The model under review builds one solid part; all positions refer to its coordinate system, in mm. Give positions to 0.01 mm unless a question says otherwise; leave off trailing zeros. Write each loop counter-clockwise with the first axis right and the second up, starting at its lowest first coordinate (ties: lowest second). Pieces come first, ordered by that corner, then holes.
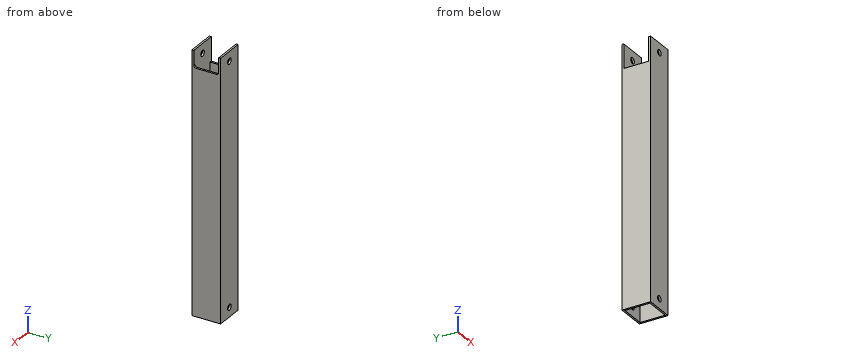
Solid Edge part; units mm, degrees
sketch "Sketch1" plane through (0, 0, 0) normal (0, 0, 1) x (1, 0, 0)
  line L0 (-81.6266, 67.336) -> (-21.6266, 67.336)
  line L1 (-21.6266, 67.336) -> (-21.6266, 127.336)
  line L2 (-21.6266, 127.336) -> (-81.6266, 127.336)
  line L3 (-81.6266, 127.336) -> (-81.6266, 67.336)
  line L4 (-77.6266, 71.336) -> (-25.6266, 71.336)
  line L5 (-25.6266, 71.336) -> (-25.6266, 123.336)
  line L6 (-25.6266, 123.336) -> (-77.6266, 123.336)
  line L7 (-77.6266, 123.336) -> (-77.6266, 71.336)
  dimension "D1" = 21.6266
  dimension "D2" = 81.6266
extrude "Protrusion1" add sketch "Sketch1" along normal blind 540
sketch "Sketch2" plane through (-56.6266, 127.336, 367.5) normal (0, 1, 0) x (0, 0, -1)
  circle A0 centre (347.5, -5) radius 6.1
  circle A1 centre (-152.5, -5) radius 6.1
extrude "Cutout1" cut sketch "Sketch2" against normal through all
sketch "Sketch3" plane through (-21.6266, 92.336, 367.5) normal (1, 0, 0) x (0, 0, -1)
  line L0 (367.49, -21) -> (367.5, -21)
  line L1 (367.5, -21) -> (367.5, 31)
  line L2 (367.5, 31) -> (367.49, 31)
  line L3 (367.49, 31) -> (367.49, -21)
  line L4 (-172.5, 31) -> (-137.5, 31)
  line L5 (-137.5, 31) -> (-137.5, -21)
  line L6 (-137.5, -21) -> (-172.5, -21)
  line L7 (-172.5, -21) -> (-172.5, 31)
  dimension "D1" = 172.5
  dimension "D2" = 137.5
  dimension "D3" = 367.49
  dimension "D4" = 367.49
extrude "Cutout2" cut sketch "Sketch3" against normal blind 5
sketch "Sketch4" plane through (-81.6266, 92.336, 367.5) normal (-1, 0, 0) x (0, 0, -1)
  line L0 (367.49, -31) -> (367.5, -31)
  line L1 (367.5, -31) -> (367.5, 21)
  line L2 (367.5, 21) -> (367.49, 21)
  line L3 (367.49, 21) -> (367.49, -31)
  line L4 (-172.5, 21) -> (-122.5, 21)
  line L5 (-122.5, 21) -> (-122.5, -31)
  line L6 (-122.5, -31) -> (-172.5, -31)
  line L7 (-172.5, -31) -> (-172.5, 21)
  dimension "D1" = 172.5
  dimension "D2" = 122.5
  dimension "D3" = 367.5
  dimension "D4" = 367.49
extrude "ExtrudedCutout_3" cut sketch "Sketch4" against normal blind 5
extrude "Cutout3" [suppressed]
fillet "Round1" radius 5 2 edges at (-23.6266, 123.336, 505) (-23.6266, 71.336, 505)
properties material "Aluminum, 6061-T6"
1) Consider section A-A, the plane x = -30.5. Give the boundary of the cut face in (y, z), then the cut area to 3 significant figures.
2) Insertion check: pin 1 (1.5 mm diameter, centred on x = -55, y = 73.5, fed in from +Z); pin 2 (1.2 mm diameter, centred on x = -80, y = 109.5, fed in from -Z); pin 3 (1.2 mm diameter, centred on x = -80.5, y = 104.5, fed in from +Z); pin 4 (2 mm diameter, centred on x = -24, y = 102, fed in from +Z). Each pin has a flat end and moves straight along its axis. Give the tip position at first contact, or say it passes through.
3) Consider section C-C, the plane y = 87. Give the boundary of the cut face in (x, z).
4) To check wall thickness, follow probe 1 along Y at (x, z) = (-37, 367.5); probe 2 along X at (y, z) = (91, 162); probe 3 along X at (y, z) = (126, 520). State the ranges of each line that lie inside material, in increasing order.
5) Consider section D-D, the plane z = 20. Give the boundary of the cut face in (x, y), then the cut area to 3 significant figures.
6) Consider section B-B, the plane z = 520. Give the boundary of the cut face in (x, y).
Answer block:
1. outline: (67.34, 0) - (71.34, 0) - (71.34, 540) - (67.34, 540) - close; (123.34, 0) - (127.34, 0) - (127.34, 540) - (123.34, 540) - close
1. area: 4,320 mm2
2. pin 1: passes through
2. pin 2: stops at z = 0.01
2. pin 3: stops at z = 490
2. pin 4: stops at z = 505
3. outline: (-81.63, 0.01) - (-77.63, 0.01) - (-77.63, 490) - (-81.63, 490) - close; (-25.63, 0.01) - (-21.63, 0.01) - (-21.63, 505) - (-25.63, 505) - close
4. probe 1: y = 67.34 to 71.34, 123.34 to 127.34
4. probe 2: x = -81.63 to -77.63, -25.63 to -21.63
4. probe 3: x = -81.63 to -57.73, -45.53 to -21.63
5. outline: (-81.63, 67.34) - (-57.73, 67.34) - (-57.73, 71.34) - (-77.63, 71.34) - (-77.63, 123.34) - (-57.73, 123.34) - (-57.73, 127.34) - (-81.63, 127.34) - close; (-45.53, 67.34) - (-21.63, 67.34) - (-21.63, 127.34) - (-45.53, 127.34) - (-45.53, 123.34) - (-25.63, 123.34) - (-25.63, 71.34) - (-45.53, 71.34) - close
5. area: 798 mm2
6. outline: (-81.63, 67.34) - (-57.73, 67.34) - (-57.73, 71.34) - (-81.63, 71.34) - close; (-81.63, 123.34) - (-57.73, 123.34) - (-57.73, 127.34) - (-81.63, 127.34) - close; (-45.53, 67.34) - (-21.63, 67.34) - (-21.63, 71.34) - (-45.53, 71.34) - close; (-45.53, 123.34) - (-21.63, 123.34) - (-21.63, 127.34) - (-45.53, 127.34) - close
